The listing builds one solid part. Answer for the finished solid, in the listing's coordinates (mm). Face numbers are marked on the shaded views. A direction names the side the tool comes from. Give positions to 0.01 mm unless a question says otherwise; leave off trailing zeros. Order: outer loops, then holes, each group sorted by start corner. A loop starts at its lowest first (then second) coordinate and runs counter-clockwise, first axis right, second up. Notation, with made-up numbers: (63, -25) - (69, -25) arc R13 cw to (69, -20) - close; hole circle Ø7 at (2.25, 81.25). An arc over 180 degrees is marked (long way). Answer as a JSON object with one key per item and string values. Group by question number.
Q1. A cutting plane is placed at C-C, the plane x = 3.75. Give the vertices of the cut face in (y, z), and give its area (3 significant figures).
Q2. Given pin 1 (3 mm diameter, centred on x = 2, z = 44.5, fed in from +Y); pin 2 (14 mm diameter, centred on y = 15, z = 20, fed in from +X); pin 3 (16.5 mm diameter, centred on y = 26.5, z = -27.5, fed in from +X), each flat-ended and moving along its own axis, determine where each tip first touches the part or whether it passes through.
Q3. Consider line 1 (Y direction, x = 4.5, z = 15.5); line 2 (Z direction, x = 2, y = 29); line 3 (X direction, y = 41.5, z = -45). Determine where each line is inside the solid, lowest interval first.
Q4. For the marked faces 1 and 2, determine the directions among +Z, -Z, +X, -X, +Y, -Y from which every point of the face is accessible in a straight line to the end or side of a thin tool.
Q5. A cutting plane is placed at A-A, the plane z = 20. Give the vertices of the cut face in (x, y), and give its area (3 significant figures).
Q6. A cutting plane is placed at B-B, the plane y = 30. Give the vertices of the cut face in (x, z), and give its area (3 significant figures).
Q7. A cutting plane is placed at D-D, the plane z = -24. Count the separate pieces of the cut face and the enclosed holes in it, and give its area (3 significant figures).
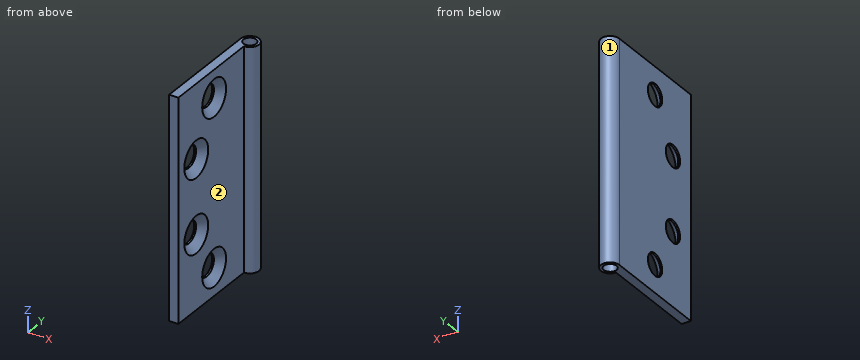
from build123d import *

# Parameters (mm, degrees)
SKETCH_1_W                  = 5
SKETCH_1_H                  = 60
EXTRUDE_2_DEPTH             = 60
SKETCH_2_R                  = 5
SKETCH_3_R                  = 3.5
CUT_EXTRUDE_1_DEPTH         = 137.839321834
HOLE_WIZARD_M101_AT_2_COUNT = 2
HOLE_WIZARD_M101_AT_2_PITCH = 29.154759474


with BuildPart() as part:
    # Эскиз1 → Вытянуть-Тонкостенный2 (new, symmetric)
    with BuildSketch(Plane.XY):
        with Locations((2.5, 30)):
            Rectangle(SKETCH_1_W, SKETCH_1_H)
    extrude(amount=EXTRUDE_2_DEPTH, both=True)

    # По траектории1: sweep along a curve in space
    with BuildLine() as sweep_1_path:
        Line((0, 60, 60), (0, 60, -60))
    # Эскиз2 → По траектории1 (sweep)
    with BuildSketch(Plane.XY.offset(60)):
        with Locations((5, 60)):
            Circle(SKETCH_2_R)
    sweep(path=sweep_1_path.line)

    # Эскиз3 → Вырез-Вытянуть1 (cut, through all)
    with BuildSketch(Plane.XY.offset(60)):
        with Locations((5, 60)):
            Circle(SKETCH_3_R)
    extrude(amount=-CUT_EXTRUDE_1_DEPTH, mode=Mode.SUBTRACT)

    # Эскиз8 → Зенковка для  винта с плоской головкой M101 (revolve, cut)
    with BuildSketch(Plane(origin=(5, 30, 45), x_dir=(0, 0, -1), z_dir=(0, 1, 0))):
        Polygon((0, 0), (0, 5), (6, 5), (6, 4), (10, 0), align=None)
    hole_wizard_m101 = revolve(axis=Axis((11.35, 30, 45), (-1, 0, 0)), mode=Mode.SUBTRACT)

    # Зенковка для  винта с плоской головкой M101 at 2: Зенковка для  винта с плоской головкой M101 ×2
    with Locations(*[Vector(0, -0.5144957554275265, -0.8574929257125442) * (i * HOLE_WIZARD_M101_AT_2_PITCH) for i in range(1, HOLE_WIZARD_M101_AT_2_COUNT)]):
        add(hole_wizard_m101, mode=Mode.SUBTRACT)

    # Зеркальное отражение1: Зенковка для  винта с плоской головкой M101 across plane
    add(hole_wizard_m101.mirror(Plane.XY), mode=Mode.SUBTRACT)

    # Зеркальное отражение1 copy 1 sketch → Зеркальное отражение1 copy 1 (revolve, cut)
    with BuildSketch(Plane(origin=(5, 15, -20), x_dir=(0, 0, 1), z_dir=(0, 1, 0))):
        Polygon((0, 0), (0, -5), (6, -5), (6, -4), (10, 0), align=None)
    revolve(axis=Axis((11.35, 15, -20), (1, 0, 0)), mode=Mode.SUBTRACT)


solid = part.part
Reply:
{
 "1": {"outline": "(0, -60) - (56.73, -60) - (56.73, 60) - (0, 60) - close; (63.27, -60) - (64.84, -60) - (64.84, 60) - (63.27, 60) - close; hole circle Ø17.5 at (15, -20); hole circle Ø17.5 at (15, 20); hole circle Ø17.5 at (30, -45); hole circle Ø17.5 at (30, 45)", "area": "6,030 mm^2"},
 "2": {"pin 1": "stops at y = 64.77", "pin 2": "stops at x = 2", "pin 3": "stops at x = 5"},
 "3": {"line 1": "y = 0 to 6.63, 23.37 to 56.54, 63.46 to 64.97", "line 2": "z = -60 to -51.93, -38.07 to 38.07, 51.93 to 60", "line 3": "x = 0 to 5"},
 "4": {"face 1": "+Z, -Z", "face 2": "+Z, -Z, +X, -Y"},
 "5": {"outline": "(0, 0) - (5, 0) - (5, 5) - (1, 9) - (0, 9) - close; (0, 21) - (1, 21) - (5, 25) - (5, 55) arc R5 ccw (long way) to (0, 60) - close; hole circle Ø7 at (5, 60)", "area": "244 mm^2"},
 "6": {"outline": "(0, -60) - (5, -60) - (5, -55) - (1, -51) - (0, -51) - close; (0, -39) - (1, -39) - (5, -35) - (5, 35) - (1, 39) - (0, 39) - close; (0, 51) - (1, 51) - (5, 55) - (5, 60) - (0, 60) - close", "area": "448 mm^2"},
 "7": {"separate pieces": "2", "enclosed holes": "1", "area": "256 mm^2"}
}
